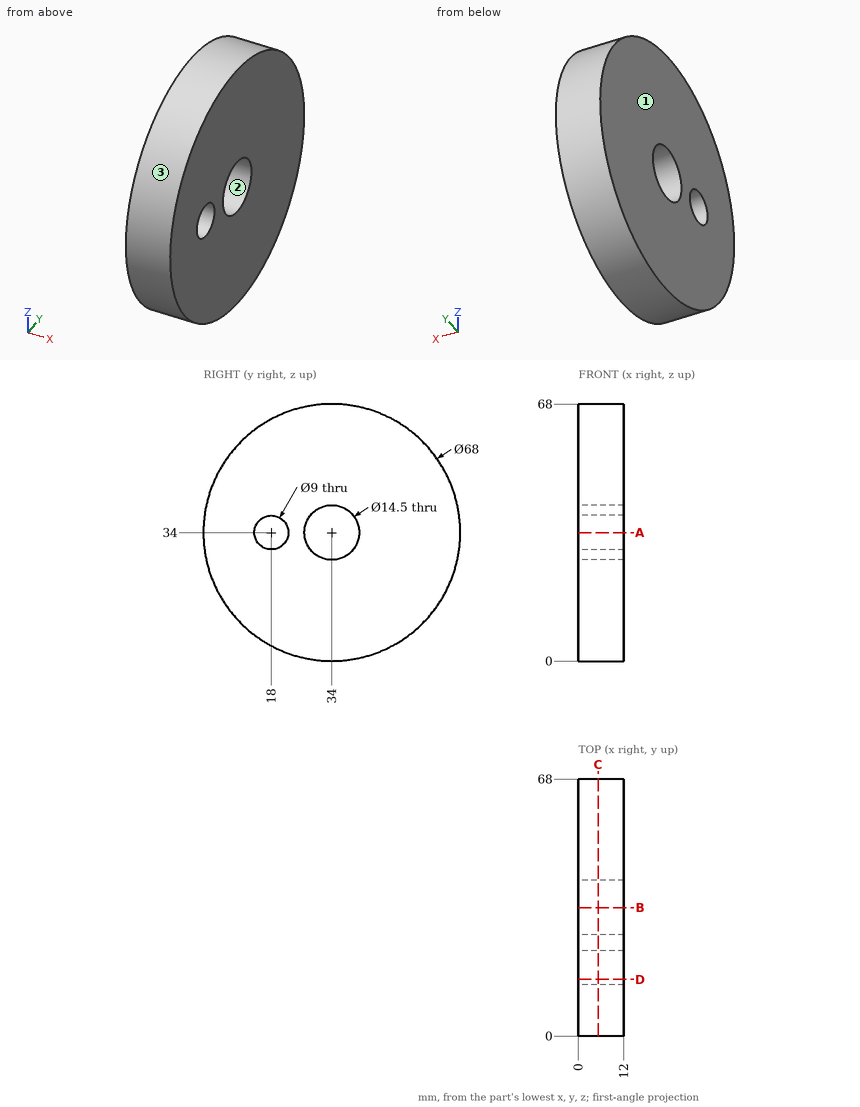
The drawing under review shows one solid part. Ordinate dimensions are in mm from its lowest x, y, z. Round coordinates to 2 decimals unless told otherwise and drop trailing zeros. Loops run counter-clockwise (first coordinate to the right, second up) from the corner with the lowest first, then second, coordinate; pieces in that order, holes last.
Item 1: Take a section at C-C (x = 5.25). Write out the cut boundary in (y, z).
Determined:
outline: circle Ø68 at (34, 34); hole circle Ø9 at (18, 34); hole circle Ø14.5 at (34, 34)
Item 2: Take a section at B-B (y = 34). Write out the cut boundary in (x, z).
Determined:
outline: (0, 0) - (12, 0) - (12, 26.75) - (0, 26.75) - close; (0, 41.25) - (12, 41.25) - (12, 68) - (0, 68) - close
Item 3: For line 1 (Y direction, x = 9.75, z = 34); line 2 (Z direction, x = 4.5, y = 38); line 3 (Z direction, x = 7, y = 27.5), list the stretches that pass through material, from the lowest coordinate up.
Determined:
line 1: y = 0 to 13.5, 22.5 to 26.75, 41.25 to 68
line 2: z = 0.24 to 27.95, 40.05 to 67.76
line 3: z = 0.63 to 30.79, 37.21 to 67.37
Item 4: Take a section at A-A (z = 34). Write out the cut boundary in (x, y), then the cut area to 3 significant figures.
Determined:
outline: (0, 0) - (12, 0) - (12, 13.5) - (0, 13.5) - close; (0, 22.5) - (12, 22.5) - (12, 26.75) - (0, 26.75) - close; (0, 41.25) - (12, 41.25) - (12, 68) - (0, 68) - close
area: 534 mm2
Item 5: Take a section at D-D (y = 15). Write out the cut boundary in (x, z).
Determined:
outline: (0, 5.8) - (12, 5.8) - (12, 30.65) - (0, 30.65) - close; (0, 37.35) - (12, 37.35) - (12, 62.2) - (0, 62.2) - close
Item 6: Mouldability with a two-part tool opening along Y and no side actions: class the marked faces 1, 2 and 3 as released by +Y, released by -Y, zero draft, split by the parting line, or undercut.
Determined:
face 1: zero draft
face 2: undercut
face 3: split by the parting line
Item 7: Clearance check with flat-ended pins moving along their axes: pin 1 Ø5 at (y, z) = (30.5, 31) entering from -X; pin 2 Ø2 at (x, y) = (8.5, 11.5) entering from -Z; pin 3 Ø4 at (x, y) = (9, 50) entering from -Z; pin 4 Ø1 at (x, z) = (3, 46) entering from -Y. State where each tip first meets the part, or that it passes through.
Determined:
pin 1: passes through
pin 2: stops at z = 7.66
pin 3: stops at z = 3.02
pin 4: stops at y = 2
